The model under review builds one solid part; all positions refer to its coordinate system, in mm. A direction names the side the tool comes from. Give positions to 0.01 mm unless a question says otherwise; leave off trailing zeros. Loops run counter-clockwise (first coordinate to the right, second up) from the corner with the lowest first, then second, coordinate; pieces in that order, holes last. Notation, with made-up numbers: M 17.25,40 L 51.25,40 A22 ccw 51.25,47 Z; hole C 72,45.25 d1. An arc over 180 degrees is marked long. One line per item, written item: value. Start each with the question number.
Q1. We need section A-A on z = -1.5. Write out the cut boundary in (x, y), plus the area to 3 significant figures.
Q2. We need section B-B on y = 2.5. Write out the cut boundary in (x, z).
Q3. We need section D-D on x = 1. Write out the cut boundary in (y, z), plus the area to 3 significant figures.
Q4. To check wall thickness, follow line 1 along X through (y, z) = (0, -1.25); line 2 along X through (y, z) = (0, 1); line 3 along X through (y, z) = (0.5, -1.75). State the ranges of each line that lie inside material, in increasing order. Write a range as from..to.
Q5. We need section C-C on x = 4.75. Write out the cut boundary in (y, z).
Q6. For pin 1 (1.6 mm diameter, centred on y = 0, z = 0, fed in from -X); pin 2 (1.7 mm diameter, centred on x = -13, y = 1, fed in from +Z); pin 3 (1.5 mm diameter, centred on y = -1.5, z = -2.5, fed in from +X); pin 4 (2 mm diameter, centred on y = 2.5, z = -1, fed in from +X), all flat-tipped, find the tip position at first contact; note any pin that passes through.
Q7. For faces 1 (the face through (8.2, 0, 1.2)), 2 (the face through (-12.46, 0.27, -0.86)), 3 (the face through (-1.63, 3.14, -1.3)), list the 3-axis set-ups (+Z, -Z, +X, -X, +Y, -Y) from which the entire face can be reached by the end or side of a thin tool; tool diameter is ignored.
Q8. Mouldability with a two-part tool opening along X and no side actions: class faces 4 (the face through (-11, 0, 2)), 5 (the face through (-12.97, -0.06, -1.95)), 6 (the face through (-3.25, 0.04, -0.05)) as released by +X, released by -X, zero draft, split by the parting line, or undercut.
```python
from build123d import *

# Parameters (mm, degrees)
M2X0_4_TAPPED_HOLE1_D           = 1.6
BOSS_EXTRUDE1_DEPTH             = 4
M2X0_4_TAPPED_HOLE2_D           = 1.6
M2X0_4_TAPPED_HOLE2_DEPTH       = 3
M2X0_4_TAPPED_HOLE2_CSINK_D     = 2.05
M2X0_4_TAPPED_HOLE2_CSINK_ANGLE = 90
M2X0_4_TAPPED_HOLE2_TIP         = 0.480688495
HOLE5_D                         = 1.8
HOLE5_DEPTH                     = 5


with BuildPart() as part:
    # Sketch1 → Revolve1 (revolve)
    with BuildSketch(Plane.XY):
        Polygon((-11, 0), (11, 0), (11, 1.95), (4.4, 1.95), (4.4, 3.4), (-7.5, 3.4), (-7.5, 4), (-11, 4), align=None)
    revolve(axis=Axis((0, 0, 0), (1, 0, 0)))

    # M2x0.4 Tapped Hole1 (through all)
    with Locations(Plane.XY.offset(3.4)):
        with Locations((-4.05, 0), (0.95, 0)):
            Hole(M2X0_4_TAPPED_HOLE1_D / 2)

    # Sketch6 → Boss-Extrude1 (add)
    with BuildSketch(Plane.ZY.offset(11)):
        with BuildLine():
            Line((0.95, 1.702938637), (0.95, -1.702938637))
            ThreePointArc((0.95, -1.702938637), (-1.95, 0), (0.95, 1.702938637))
        make_face()
    extrude(amount=BOSS_EXTRUDE1_DEPTH)

    # M2x0.4 Tapped Hole2
    with Locations(Plane.XY.offset(3.4)):
        with Locations((7.4, 0)):
            CounterSinkHole(M2X0_4_TAPPED_HOLE2_D / 2, M2X0_4_TAPPED_HOLE2_CSINK_D / 2, depth=M2X0_4_TAPPED_HOLE2_DEPTH, counter_sink_angle=M2X0_4_TAPPED_HOLE2_CSINK_ANGLE)
            with Locations((0, 0, -(M2X0_4_TAPPED_HOLE2_DEPTH + M2X0_4_TAPPED_HOLE2_TIP / 2))):  # 118° drill point
                Cone(0, M2X0_4_TAPPED_HOLE2_D / 2, M2X0_4_TAPPED_HOLE2_TIP, mode=Mode.SUBTRACT)

    # Hole5
    with Locations(Plane.ZY.offset(15)):
        with Locations((0, 0)):
            Hole(HOLE5_D / 2, depth=HOLE5_DEPTH)


solid = part.part
```
Solved:
1. outline: M -15,-1.25 L -11,-1.25 L -11,-3.71 L -7.5,-3.71 L -7.5,-3.05 L 4.4,-3.05 L 4.4,-1.25 L 11,-1.25 L 11,1.25 L 4.4,1.25 L 4.4,3.05 L -7.5,3.05 L -7.5,3.71 L -11,3.71 L -11,1.25 L -15,1.25 Z; hole C -4.05,0 d1.6; hole C 0.95,0 d1.6
1. area: 121 mm2
2. outline: M -11,-3.12 L -7.5,-3.12 L -7.5,-2.3 L 4.4,-2.3 L 4.4,2.3 L -7.5,2.3 L -7.5,3.12 L -11,3.12 Z
3. outline: M -0.8,-3.3 L -0.8,3.3 A3.4 ccw Z; M 0.8,-3.3 A3.4 ccw 0.8,3.3 Z
3. area: 25.6 mm2
4. line 1: -15..-4.85, -3.25..0.15, 1.75..11
4. line 2: -11..-4.85, -3.25..0.15, 1.75..6.6, 8.2..11
4. line 3: -15..-4.67, -3.43..0.33, 1.57..11
5. outline: C 0,0 d3.9
6. pin 1: x = -10
6. pin 2: z = 0.95
6. pin 3: x = 4.4
6. pin 4: x = 11
7. face 1: +Z
7. face 2: -X
7. face 3: +X
8. face 4: released by -X
8. face 5: zero draft
8. face 6: undercut
